Check sheet for the drawn part. Datum: minimum x, y, z corner. Units: mm. A direction names the side the tool comes from. Coordinates: 2 decimals unless noted, no trailing zeros. Write each loop counter-clockwise with the first axis right and the second up, starting at its lowest first coordinate (ties: lowest second). Pieces come first, ordered by that corner, then holes. Notation, with made-up numbers: M 78,43.25 L 104,43.25 A19 cw 104,70.25 Z; hole C 28,22.5 d7. An arc over 180 degrees is marked long. Write item = value, one per line. Start each with the question number.
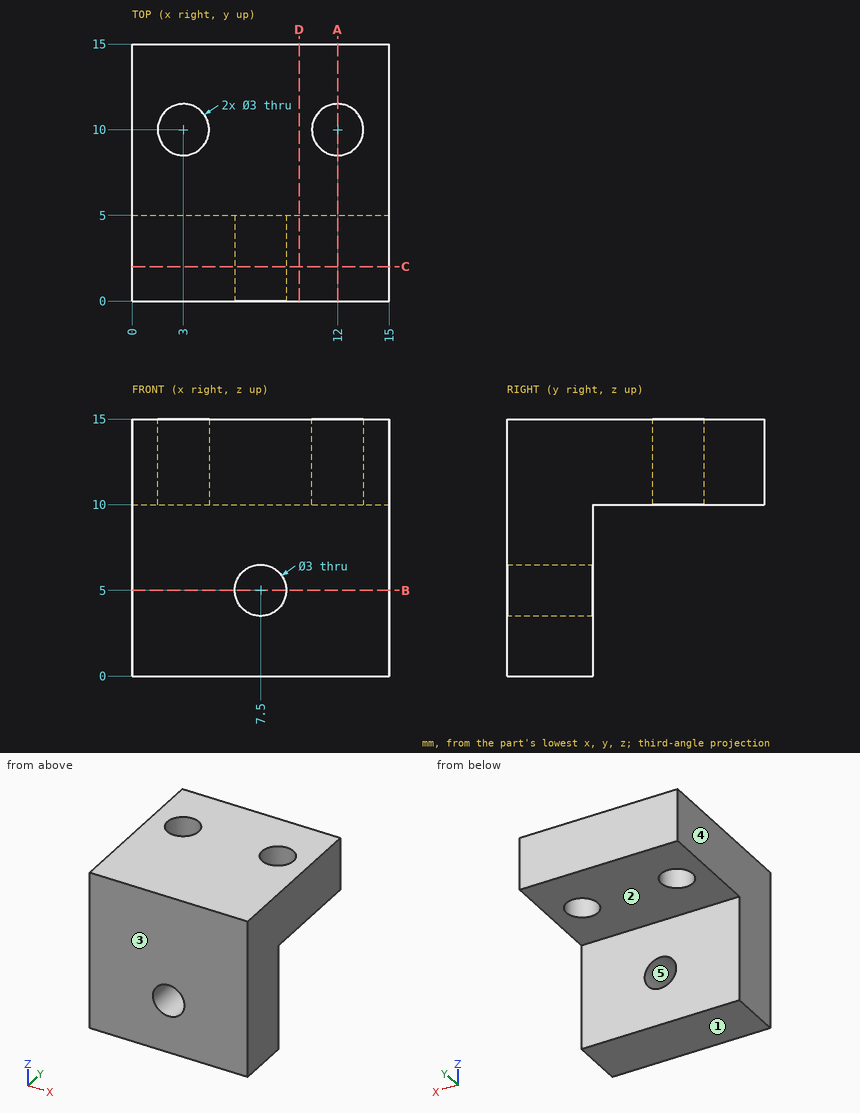
Q1. Gauge pin test, flat ends, axial feed: pin 1 (6 mm diameter, centred on y = 6.5, z = 8.5, fed in from -X); pin 2 (5 mm diameter, centred on x = 4.5, z = 4.5, fed in from +Y); pin 3 (2.5 mm diameter, centred on x = 7.5, z = 5, fed in from +Y); pin 4 (3 mm diameter, centred on x = 4.5, y = 9, fed in from -Z). Record the tip position at first contact, or that the pin passes through.
Q2. Cross-section at D-D on x = 9.75. Enter the section's corners in (y, z), and give its area (3 significant figures).
Q3. Scan lines: L1, parallel to Y at x = 3, z = 13.65; L2, parallel to X at y = 3.9, z = 5; L3, parallel to Y at x = 2.75, z = 5.75. Record each from-to range of solid material in increasing order.
Q4. Draft check along X on the marked faces 3, 4 and 5. Enter one of: pulls with the +X half, pulls with the -X half, needs draft (parallel to the pull), parting line crosses it, or undercut.
Q5. Set-up check for the marked faces 1 and 2: record each of +Z, -Z, +X, -X, +Y, -Y from which the full face is reachable in a straight line by a thin tool's end or side.
Q6. Cross-section at A-A on x = 12. Enter the section's corners in (y, z), and give its area (3 significant figures).
Q7. Cross-section at C-C on y = 2. Enter the section's corners in (x, z).
Q8. Cross-section at B-B on z = 5. Enter the section's corners in (x, y).
Values found:
q1.pin_1 = 0
q1.pin_2 = 5
q1.pin_3 = through
q1.pin_4 = 10
q2.outline = M 0,0 L 5,0 L 5,10 L 15,10 L 15,15 L 0,15 Z
q2.area = 125 mm²
q3.L1 = 0 to 8.5, 11.5 to 15
q3.L2 = 0 to 6, 9 to 15
q3.L3 = 0 to 5
q4.face_3 = needs draft
q4.face_4 = pulls with the -X half
q4.face_5 = undercut
q5.face_1 = -Z, +X, -X, +Y, -Y
q5.face_2 = -Z, +X, -X, +Y
q6.outline = M 0,0 L 5,0 L 5,10 L 8.5,10 L 8.5,15 L 0,15 Z; M 11.5,10 L 15,10 L 15,15 L 11.5,15 Z
q6.area = 110 mm²
q7.outline = M 0,0 L 15,0 L 15,15 L 0,15 Z; hole C 7.5,5 d3
q8.outline = M 0,0 L 6,0 L 6,5 L 0,5 Z; M 9,0 L 15,0 L 15,5 L 9,5 Z
